from build123d import *

# Parameters (mm, degrees)
F1_DEPTH = 50
F2_W     = 25
F2_H     = 17
F3_DEPTH = 2


with BuildPart() as f1:
    # F0 (on Front) → F1 (new body)
    with BuildSketch(Plane.XZ):
        with BuildLine():
            Line((0, 14.117118), (0, 0))
            Line((0, 0), (25, 0))
            Line((25, 0), (25, 14.117118))
            ThreePointArc((25, 14.117118), (23.98797, 19.044242), (21.115752, 23.173542))
            ThreePointArc((21.115752, 23.173542), (20.161384, 23.785734), (19.047972, 24))
            Line((19.047972, 24), (18.98802, 24))
            ThreePointArc((18.98802, 24), (18.037353, 23.310214), (18.3982, 22.192465))
            ThreePointArc((18.3982, 22.192465), (12.5, 4.117118), (6.6018, 22.192465))
            ThreePointArc((6.6018, 22.192465), (6.962647, 23.310214), (6.01198, 24))
            Line((6.01198, 24), (5.952028, 24))
            ThreePointArc((5.952028, 24), (4.838616, 23.785734), (3.884248, 23.173542))
            ThreePointArc((3.884248, 23.173542), (1.01203, 19.044242), (0, 14.117118))
        make_face()
    extrude(amount=F1_DEPTH)

    # F2 (on face) → F3 (join)
    with BuildSketch(Plane(origin=(0, 0, 0), x_dir=(1, 0, 0), z_dir=(0, 0, -1))):
        with Locations((12.5, 44.5)):
            Rectangle(F2_W, F2_H)
    extrude(amount=F3_DEPTH)


solid = f1.part
Verification items for the finished model (mm, model axes). A direction names the side the tool comes from. Coordinates: 2 decimals unless noted, no trailing zeros. Write each loop counter-clockwise with the first axis right and the second up, starting at its lowest first coordinate (ties: lowest second). Pieces come first, ordered by that corner, then holes. Notation, with made-up numbers: (-9, 21) -> (26, 21) arc R23 ccw to (26, 33) -> close; hole circle Ø6 at (68, -12.75). An arc over 180 degrees is marked (long way). One line per item, written item: value. Start each with the question number.
Q1. Cross-section at B-B on z = 9.75. Enter the section's corners in (x, y).
Q2. Cross-section at D-D on y = -39. Enter the section's corners in (x, z), and give its area (3 significant figures).
Q3. Cross-section at C-C on x = 3.25. Enter the section's corners in (y, z), and give its area (3 significant figures).
Q4. Go/stop test with flat-tipped pins: P1, Ø1, axis at x = 2.5, z = 5.5, coming from the -Y side; P2, Ø1.5, axis at x = 16.5, y = -31, coming from the -Z side; P3, Ø0.9, axis at x = 18.5, y = -52, coming from the +Z side. Record where each tip stops, or that it passes through.
Q5. Mould release check, pull along X, two halves, no side actions. Record for faces 5 (the flat face through (12, -45, -2)), 6 (the cylindrical face through (18.043, -24.65, 23.327)), 7 (the cylindrical face through (4.85, -24.65, 23.79)): pulls with the +X half, pulls with the -X half, needs draft (parallel to the pull), parting line crosses it, or undercut.
Q6. Thickness scan on L1, parallel to X at y = -16, z = 6.5; L2, parallel to X at y = -38, z = 11.75; L3, parallel to Z at x = 12.5, y = -33.5. Record the ranges inside material, lowest first. Write a range as from..to.
Q7. Cross-section at A-A on x = 12.5. Enter the section's corners in (y, z).
Q8. Access from +Z, -Z, +X, -X, +Y, -Y to the whole of each face (thin tool, end or side, straight path). Record for faces 1 (the flat face through (12, -52, 0)), 2 (the flat face through (0, -26, 6)), 3 (the flat face through (12, -18, 0)), 4 (the cylindrical face through (6.97, -24.65, 23.29)).
Checked values:
1. outline: (0, -50) -> (3.5, -50) -> (3.5, 0) -> (0, 0) -> close; (21.5, -50) -> (25, -50) -> (25, 0) -> (21.5, 0) -> close
2. outline: (0, -2) -> (25, -2) -> (25, 14.12) arc R12.5 ccw to (21.12, 23.17) arc R3 ccw to (19.05, 24) -> (18.99, 24) arc R1 ccw to (18.4, 22.19) arc R10 cw (long way) to (6.6, 22.19) arc R1 ccw to (6.01, 24) -> (5.95, 24) arc R3 ccw to (3.88, 23.17) arc R12.5 ccw to (0, 14.12) -> close
2. area: 302 mm²
3. outline: (-53, -2) -> (-36, -2) -> (-36, 0) -> (0, 0) -> (0, 10.32) -> (-50, 10.32) -> (-50, 0) -> (-53, 0) -> close; (-50, 17.92) -> (0, 17.92) -> (0, 22.52) -> (-50, 22.52) -> close
3. area: 780 mm²
4. P1: stops at y = -50
4. P2: stops at z = 0
4. P3: stops at z = 0
5. face 5: needs draft
5. face 6: undercut
5. face 7: pulls with the -X half
6. L1: x = 0..6.02, 18.98..25
6. L2: x = 0..2.78, 22.22..25
6. L3: z = 0..4.12
7. outline: (-53, -2) -> (-36, -2) -> (-36, 0) -> (0, 0) -> (0, 4.12) -> (-50, 4.12) -> (-50, 0) -> (-53, 0) -> close
8. face 1: +Z, +X, -X, -Y
8. face 2: +Z, -Z, -X, +Y, -Y
8. face 3: -Z, +X, -X, +Y
8. face 4: +Y, -Y
